Build history of the part. All positions in model axes, mm. Give positions to 0.01 mm unless a question says otherwise; leave off trailing zeros. Write each loop counter-clockwise with the first axis right and the second up, starting at its lowest first coordinate (ties: lowest second). Pieces come first, ordered by that corner, then holes. Notation, with made-up numbers: (39, 82.25) -> (59, 82.25) arc R13 ccw to (59, 88.25) -> close; hole circle Ø9 at (35.25, 5). An arc over 180 degrees is marked (long way). One line per question, with ' | ' between items. Start each with the question number.
(1) Drill centre lines: probe 1 along X at (y, z) = (50, 2.85); probe 2 along X at (y, z) = (-72.5, 0.3); probe 3 along Y at (x, z) = (96.5, 4). Where is each one in solid material? Low to high. Write a range as from..to.
(2) Band-saw the part on C-C, the plane z = 1.65. Count the separate pieces of the cut face and the enclosed holes in it, and give its area (3 significant figures).
(3) Band-saw the part on B-B, the plane x = 22.5. Give the cut face in (y, z), and give its area (3 significant figures).
(4) Pin check, flat tips, straight feed: P1, Ø2, axis at y = -30.5, z = 1, coming from the +X side; P2, Ø3, axis at x = -17, z = 3, coming from the +Y side; P3, Ø2.5, axis at x = 96.5, y = 0, coming from the -Z side; P4, Ø1.5, axis at x = -85.5, z = 2, coming from the +Y side. Stop position of each tip, or through.
(5) Band-saw the part on A-A, the plane x = -33. Give the cut face in (y, z), and give its area (3 significant figures).
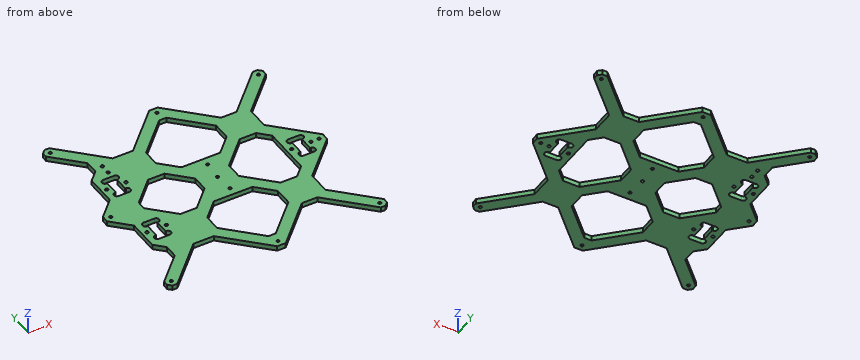
from build123d import *

# Parameters (mm, degrees)
PAD_DEPTH       = 5
SKETCH001_R     = 1.5
POCKET_DEPTH    = 5
SKETCH002_R     = 1.6
POCKET001_DEPTH = 510.471078
SKETCH003_R     = 1.6
POCKET002_DEPTH = 5.001


with BuildPart() as part:
    # Sketch → Pad (new body)
    with BuildSketch(Plane.XY):
        Polygon((-116, 0), (-116, 3.664466), (-98.5, 21.164466), (-98.5, 52.5), (-89, 62), (-89, 75.464466), (-116, 102.464466), (-116, 107.464466), (-112.464466, 111), (-107.464466, 111), (-66.464466, 70), (-45.4, 70), (-4.4, 111), (4.4, 111), (45.4, 70), (61.464466, 70), (102.464466, 111), (107.464466, 111), (111, 107.464466), (111, 102.464466), (73, 64.464466), (73, 41.664466), (111, 3.664466), (111, 0), align=None)
    pad = extrude(amount=PAD_DEPTH)

    # Sketch001 → Pocket (cut)
    with BuildSketch(Plane.XY.offset(5)):
        with Locations((-110, 0)):
            Circle(SKETCH001_R)
        with Locations((-110, 105)):
            Circle(SKETCH001_R)
        with Locations((0, 105)):
            Circle(SKETCH001_R)
        with Locations((105, 105)):
            Circle(SKETCH001_R)
        with Locations((105, 0)):
            Circle(SKETCH001_R)
        Circle(SKETCH001_R)
        with Locations((1.5, 19.5)):
            Circle(SKETCH001_R)
        Polygon((-78.5, 0), (-78.5, 4.5), (-55, 28), (-38, 28), (-18, 8), (-18, 0), align=None)
        Polygon((17, 0), (17, 8.5), (44, 35.5), (61, 35.5), (71.5, 25), (71.5, 0), align=None)
        Polygon((-3.75, 94.75), (3.75, 94.75), (36, 62.5), (36, 44.5), (19.5, 28), (-20.5, 28), (-37, 44.5), (-37, 61.5), align=None)
    pocket = extrude(amount=-POCKET_DEPTH, mode=Mode.SUBTRACT)

    # Sketch002 → Pocket001 (cut, through all)
    with BuildSketch(Plane.XY.offset(5)):
        with Locations((-93.5, 35)):
            Circle(SKETCH002_R)
        with Locations((-73.5, 35)):
            Circle(SKETCH002_R)
        with Locations((76.5, 0)):
            Circle(SKETCH002_R)
        with Locations((96.5, 0)):
            Circle(SKETCH002_R)
        with BuildLine():
            ThreePointArc((-89.1, 48.25), (-92.1, 45.25), (-89.1, 42.25))
            Line((-89.1, 42.25), (-89, 42.25))
            Line((-89, 42.25), (-88.5, 41.75))
            Line((-88.5, 41.75), (-88.5, 28.25))
            Line((-88.5, 28.25), (-89, 27.75))
            Line((-89, 27.75), (-89.1, 27.75))
            ThreePointArc((-89.1, 27.75), (-92.1, 24.75), (-89.1, 21.75))
            Line((-89.1, 21.75), (-77.9, 21.75))
            ThreePointArc((-77.9, 21.75), (-74.9, 24.75), (-77.9, 27.75))
            Line((-77.9, 27.75), (-78, 27.75))
            Line((-78, 27.75), (-78.5, 28.25))
            Line((-78.5, 28.25), (-78.5, 41.75))
            Line((-78.5, 41.75), (-78, 42.25))
            Line((-78, 42.25), (-77.9, 42.25))
            ThreePointArc((-77.9, 42.25), (-74.9, 45.25), (-77.9, 48.25))
            Line((-77.9, 48.25), (-89.1, 48.25))
        make_face()
        with BuildLine():
            ThreePointArc((80.9, 13.25), (77.9, 10.25), (80.9, 7.25))
            Line((80.9, 7.25), (81, 7.25))
            Line((81, 7.25), (81.5, 6.75))
            Line((81.5, 6.75), (81.5, 0))
            Line((81.5, 0), (91.5, 0))
            Line((91.5, 0), (91.5, 6.75))
            Line((91.5, 6.75), (92, 7.25))
            Line((92, 7.25), (92.1, 7.25))
            ThreePointArc((92.1, 7.25), (95.1, 10.25), (92.1, 13.25))
            Line((92.1, 13.25), (80.9, 13.25))
        make_face()
    pocket001 = extrude(amount=-POCKET001_DEPTH, mode=Mode.SUBTRACT)

    # Mirrored: Pad, Pocket, Pocket001 across Sketch H_Axis
    add(pad.mirror(Plane.ZX))
    add(pocket.mirror(Plane.ZX), mode=Mode.SUBTRACT)
    add(pocket001.mirror(Plane.ZX), mode=Mode.SUBTRACT)

    # Sketch003 → Pocket002 (cut, through all)
    with BuildSketch(Plane.XY.offset(5)):
        with Locations((-80, 65)):
            Circle(SKETCH003_R)
        with Locations((-80, 55)):
            Circle(SKETCH003_R)
    extrude(amount=-POCKET002_DEPTH, mode=Mode.SUBTRACT)


solid = part.part
Results:
1) probe 1: x = -98.5..-37, 36..73 | probe 2: x = -89..-68.96, -42.9..-26, 26..42.9, 63.96..81.04 | probe 3: y = -105.04..-87.96, -18.16..-1.6, 1.6..18.16, 87.96..105.04
2) separate pieces: 1 | enclosed holes: 26 | area: 19,000 mm²
3) outline: (-92.9, 0) -> (-76, 0) -> (-76, 5) -> (-92.9, 5) -> close; (-31, 0) -> (-14, 0) -> (-14, 5) -> (-31, 5) -> close; (14, 0) -> (31, 0) -> (31, 5) -> (14, 5) -> close; (76, 0) -> (92.9, 0) -> (92.9, 5) -> (76, 5) -> close | area: 339 mm²
4) P1: stops at x = 85.16 | P2: stops at y = 99.9 | P3: passes through | P4: stops at y = 89.79
5) outline: (-82.4, 0) -> (-65.5, 0) -> (-65.5, 5) -> (-82.4, 5) -> close; (-40.5, 0) -> (-23, 0) -> (-23, 5) -> (-40.5, 5) -> close; (23, 0) -> (40.5, 0) -> (40.5, 5) -> (23, 5) -> close; (65.5, 0) -> (82.4, 0) -> (82.4, 5) -> (65.5, 5) -> close | area: 344 mm²
